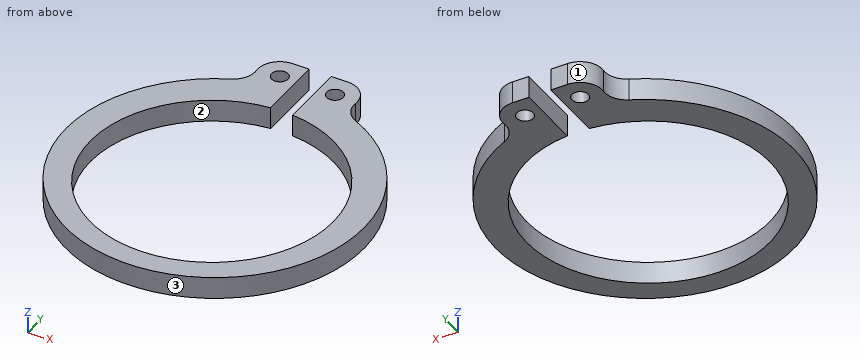
```python
from build123d import *

# Parameters (mm, degrees)
IZIM1_R                     = 0.75
Y_KSEKLIK_EKSTR_ZYON1_DEPTH = 1


with BuildPart() as part:
    # Çizim1 → Yükseklik-Ekstrüzyon1 (new body, symmetric)
    with BuildSketch(Plane.XY):
        with BuildLine():
            Line((-2.5, 16.498872216), (-1, 16.498872216))
            Line((-1, 16.498872216), (-1, 10.45445115))
            ThreePointArc((-1, 10.45445115), (0, -11.5), (1, 10.45445115))
            Line((1, 10.45445115), (1, 16.498872216))
            Line((1, 16.498872216), (2.5, 16.498872216))
            ThreePointArc((2.5, 16.498872216), (3.985473902, 15.837481746), (4.487915198, 14.290994496))
            ThreePointArc((4.487915198, 14.290994496), (4.738807919, 13.092499976), (5.641216256, 12.264855448))
            ThreePointArc((5.641216256, 12.264855448), (0, -13.5), (-5.641216256, 12.264855448))
            ThreePointArc((-5.641216256, 12.264855448), (-4.738807919, 13.092499976), (-4.487915198, 14.290994496))
            ThreePointArc((-4.487915198, 14.290994496), (-3.985473902, 15.837481746), (-2.5, 16.498872216))
        make_face()
        with Locations((-2.5, 14.5)):
            Circle(IZIM1_R, mode=Mode.SUBTRACT)
        with Locations((2.5, 14.5)):
            Circle(IZIM1_R, mode=Mode.SUBTRACT)
    extrude(amount=Y_KSEKLIK_EKSTR_ZYON1_DEPTH, both=True)


solid = part.part
```
For this review, take the finished solid that the model builds, in its own axes (mm). Face numbers are marked on the shaded views. Coordinates: 2 decimals unless noted, no trailing zeros. Loops run counter-clockwise (first coordinate to the right, second up) from the corner with the lowest first, then second, coordinate; pieces in that order, holes last. Notation, with made-up numbers: (66, 23) - (85, 23) arc R27 ccw to (85, 53) - close; hole circle Ø2 at (37.25, 22). An arc over 180 degrees is marked (long way). Use one line per item in the form item = value. Start each with the question number.
1) Take a section at B-B (x = 4). State the section outline as (y, z) points.
2) Draft analysis for pull direction X (two halves, no side actions). For the marked faces 1, 2 and 3, state which applies: released by +X, released by -X, zero draft, split by the parting line, or undercut.
3) Take a section at C-C (z = -0.1). State the section outline as (x, y) points.
4) Take a section at A-A (y = -2.5). State the section outline as (x, z) points, plus the area to 3 significant figures.
5) For pin 1 (0.6 mm diameter, centred on y = 12.5, z = 0.5, fed in from -X); pin 2 (8 mm diameter, centred on x = -3, y = -2.5, fed in from +Z); pin 3 (2.5 mm diameter, centred on x = -2.5, y = 14.5, fed in from -Z); pin 4 (0.6 mm diameter, centred on y = 14.5, z = 0.5, fed in from +X), all flat-tipped, find the tip position at first contact; note any pin that passes through.
6) To check wall thickness, follow probe 1 along Y at (x, z) = (-2.5, 0.9); probe 2 along X at (y, z) = (13.5, -0.75); probe 3 along Y at (x, z) = (-4, 0.2). State the ranges of each line that lie inside material, in increasing order. Write a range as from..to.
7) Take a section at D-D (x = 0). State the section outline as (y, z) points.
From the geometry:
q1.outline = (-12.89, -1) - (-10.75, -1) - (-10.75, 1) - (-12.89, 1) - close; (9.75, -1) - (15.82, -1) - (15.82, 1) - (9.75, 1) - close
q2.face_1 = released by -X
q2.face_2 = undercut
q2.face_3 = split by the parting line
q3.outline = (-5.64, 12.26) arc R13.5 ccw (long way) to (5.64, 12.26) arc R2 cw to (4.49, 14.29) arc R2 ccw to (2.5, 16.5) - (1, 16.5) - (1, 10.45) arc R11 cw (long way) to (-1, 10.45) - (-1, 16.5) - (-2.5, 16.5) arc R2 ccw to (-4.49, 14.29) arc R2 cw to start; hole circle Ø1.5 at (-2.5, 14.5); hole circle Ø1.5 at (2.5, 14.5)
q4.outline = (-13.27, -1) - (-10.82, -1) - (-10.82, 1) - (-13.27, 1) - close; (10.82, -1) - (13.27, -1) - (13.27, 1) - (10.82, 1) - close
q4.area = 9.80 mm2
q5.pin_1 = -5.78
q5.pin_2 = through
q5.pin_3 = -1
q5.pin_4 = 4.5
q6.probe_1 = -13.27..-11.21, 10.21..13.75, 15.25..16.5
q6.probe_2 = -4.56..-1, 1..4.56
q6.probe_3 = -12.89..-10.75, 9.75..15.82
q7.outline = (-13.5, -1) - (-11.5, -1) - (-11.5, 1) - (-13.5, 1) - close
